The listing builds one solid part. Answer for the finished solid, in the listing's coordinates (mm). Face numbers are marked on the shaded views. A direction names the side the tool comes from. Round coordinates to 2 decimals unless told otherwise and drop trailing zeros. Write each loop counter-clockwise with the first axis right and the second up, starting at its lowest first coordinate (ties: lowest second). Pieces come first, ordered by that corner, then holes. Notation, with made-up numbers: (9.25, 53.5) - (19.25, 53.5) arc R22 ccw to (19.25, 69.5) - close; hole circle Ø4 at (31, 64). An arc over 180 degrees is marked (long way). Answer as CSV lines item,"result". Start each with the question number.
Item 1: Straight lines are drawn through the part: line 1 along X through (y, z) = (16.47, 1.3) (3 decimals); line 2 along X through (y, z) = (14.75, -0.85); line 3 along X through (y, z) = (15.75, 0.85). For each, find the intervals that lie inside material, in ascending order. Write a range as [from, to].
Item 2: Which of the six approach directions +Z, -Z, +X, -X, +Y, -Y give full straight-line access (tool end or side, diameter ignored) to the marked faces 5 and 6?
Item 3: Flat-ended cylindrical pins translate along their axes: pin 1 (12 mm diameter, centred on x = 1.5, y = 15, fed in from -Z); pin 2 (1 mm diameter, centred on y = 15, z = 2, fed in from -X); pin 3 (1.5 mm diameter, centred on y = 1.5, z = -0.5, fed in from -X). Find the tip coordinate at first contact, or state that the pin passes through.
Item 4: A cutting plane is placed at B-B on z = 2.35. Determine the outline of the cut face in (x, y) (3 decimals), and give its area (3 significant figures).
Item 5: A cutting plane is placed at C-C on y = 16.47. State how many separate pieces and enclosed holes the cut face has, and give its area (3 significant figures).
Item 6: For a pull along X with two mould halves and no side action, classify the marked faces 1, 2, 3 and 4 as pulls with the +X half, pulls with the -X half, needs draft (parallel to the pull), parting line crosses it, or undercut.
```python
from build123d import *
from build123d.topology import SkipClean

# Parameters (mm, degrees)
SKETCH1_R           = 2.0500000000000003
SKETCH1_R_2         = 2.05
BOSS_EXTRUDE1_DEPTH = 3
BOSS_EXTRUDE2_START = 2.95
SKETCH2_R           = 4.999999999999997
SKETCH2_R_2         = 2.05
SKETCH2_R_3         = 4.999999999999999
SKETCH2_R_4         = 2.0500000000000003
SKETCH2_R_5         = 4.999999999999998
SKETCH2_R_6         = 2.0499999999999985
BOSS_EXTRUDE2_DEPTH = 2.95
CHAMFER1_SIZE       = 2.95
SKETCH3_W           = 37.85330439531782
SKETCH3_H           = 28.758532039103056
CUT_EXTRUDE1_DEPTH  = 0.5


with BuildPart() as part:
    # Sketch1 → Boss-Extrude1 (new body)
    with BuildSketch(Plane.XY):
        with BuildLine():
            Line((-14.411027514700965, 13.845837315616981), (-4.256027514700967, -2.624162684383019))
            ThreePointArc((-4.256027514700967, -2.624162684383019), (3.1e-16, -4.999999999999998), (4.256027514700967, -2.624162684383019))
            Line((4.256027514700967, -2.624162684383019), (14.411027514700965, 13.845837315616981))
            ThreePointArc((14.411027514700965, 13.845837315616981), (14.52082256979799, 18.907128082198888), (10.155000000000001, 21.46999999999999))
            Line((10.155000000000001, 21.46999999999999), (-10.155000000000001, 21.46999999999999))
            ThreePointArc((-10.155000000000001, 21.46999999999999), (-14.520822569797986, 18.907128082198888), (-14.411027514700965, 13.845837315616981))
        make_face()
        with Locations((-10.155, 16.47)):
            Circle(SKETCH1_R, mode=Mode.SUBTRACT)
        with Locations((10.155, 16.47)):
            Circle(SKETCH1_R, mode=Mode.SUBTRACT)
        Circle(SKETCH1_R_2, mode=Mode.SUBTRACT)
    extrude(amount=BOSS_EXTRUDE1_DEPTH)

    # Sketch2 → Boss-Extrude2 (add)
    # profile 1 of 3: a face of its own
    with BuildSketch(Plane(origin=(0, 0, 0), x_dir=(-1, 0, 0), z_dir=(0, 0, -1)).offset(BOSS_EXTRUDE2_START)):
        Circle(SKETCH2_R)
        Circle(SKETCH2_R_2, mode=Mode.SUBTRACT)
    # profile 2 of 3: a face of its own
    with BuildSketch(Plane(origin=(0, 0, 0), x_dir=(-1, 0, 0), z_dir=(0, 0, -1)).offset(BOSS_EXTRUDE2_START)):
        with Locations((10.155, 16.47)):
            Circle(SKETCH2_R_3)
        with Locations((10.155, 16.47)):
            Circle(SKETCH2_R_4, mode=Mode.SUBTRACT)
    # profile 3 of 3: a face of its own
    with BuildSketch(Plane(origin=(0, 0, 0), x_dir=(-1, 0, 0), z_dir=(0, 0, -1)).offset(BOSS_EXTRUDE2_START)):
        with Locations((-10.155, 16.47)):
            Circle(SKETCH2_R_5)
        with Locations((-10.155, 16.47)):
            Circle(SKETCH2_R_6, mode=Mode.SUBTRACT)
    extrude(amount=-BOSS_EXTRUDE2_DEPTH)

    # Chamfer1
    chamfer1_edges = [part.edges().sort_by_distance(p)[0] for p in [
        (4.999999999999997, 6.1e-16, -2.95),
        (-5.155, 16.47, -2.95),
        (15.154999999999998, 16.47, -2.95),
    ]]
    chamfer(chamfer1_edges, length=CHAMFER1_SIZE - 0.0001)  # a hair under: the kernel refuses the full size

    # Sketch3 → Cut-Extrude1 (cut)
    with SkipClean():  # the faces are left unmerged after this step: merging them gives an invalid solid
        with BuildSketch(Plane.XY.offset(-2.95)):
            with Locations((0.24948253346224725, 7.962837236222983)):
                Rectangle(SKETCH3_W, SKETCH3_H)
        extrude(amount=CUT_EXTRUDE1_DEPTH, mode=Mode.SUBTRACT)


solid = part.part
```
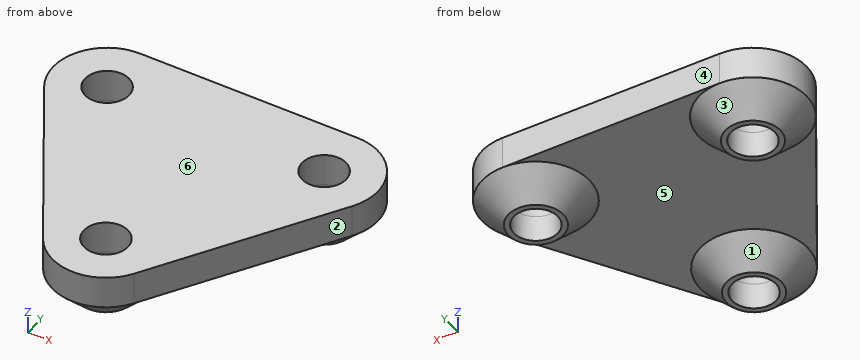
Geometry says:
1,line 1,"x = [-15.155, -12.205], [-8.105, 8.105], [12.205, 15.155]"
1,line 2,"x = [-13.93, -11.27], [-9.04, -6.38], [6.38, 9.04], [11.27, 13.93]"
1,line 3,"x = [-15.1, -12.07], [-8.24, 8.24], [12.07, 15.1]"
2,face 5,"-Z"
2,face 6,"+Z, +X, -X, +Y, -Y"
3,pin 1,"stops at z = -2.22"
3,pin 2,"stops at x = -15.06"
3,pin 3,"stops at x = -7.14"
4,outline,"(-14.411, 13.846) - (-4.256, -2.624) arc R5 ccw to (4.256, -2.624) - (14.411, 13.846) arc R5 ccw to (10.155, 21.47) - (-10.155, 21.47) arc R5 ccw to start; hole circle Ø4.1 at (-10.155, 16.47); hole circle Ø4.1 at (0, 0); hole circle Ø4.1 at (10.155, 16.47)"
4,area,"501 mm^2"
5,separate pieces,"3"
5,enclosed holes,"0"
5,area,"83.2 mm^2"
6,face 1,"parting line crosses it"
6,face 2,"pulls with the +X half"
6,face 3,"undercut"
6,face 4,"needs draft"
